Design review of the part built by this model. Coordinates are the model's own, in mm. A direction names the side the tool comes from. Coordinates: 2 decimals unless noted, no trailing zeros. Loops run counter-clockwise (first coordinate to the right, second up) from the corner with the lowest first, then second, coordinate; pieces in that order, holes last. Notation, with made-up numbers: (53, 54.5) - (105, 54.5) arc R22 cw to (105, 81.5) - close; hole circle Ø6 at (-34.5, 65.25). An arc over 180 degrees is marked (long way). One line per question, with ' | ' between items.
from build123d import *

# Parameters (mm, degrees)
SKETCH1_R           = 40
BOSS_EXTRUDE1_DEPTH = 4
SKETCH8_R           = 5
BOSS_EXTRUDE3_DEPTH = 5


with BuildPart() as part:
    # Sketch1 → Boss-Extrude1 (new body, symmetric)
    with BuildSketch(Plane(origin=(0, 0, 0), x_dir=(1, 0, 0), z_dir=(0, 1, 0))):
        Circle(SKETCH1_R)
    extrude(amount=BOSS_EXTRUDE1_DEPTH, both=True)

    # Sketch8 → Boss-Extrude3 (add)
    with BuildSketch(Plane(origin=(0, 0, 0), x_dir=(0, 0, -1), z_dir=(1, 0, 0))):
        with BuildLine():
            Line((0, 4), (-30, 4))
            Line((-30, 4), (37.824592442, 80.62784488))
            ThreePointArc((37.824592442, 80.62784488), (50.453649811, 82.577329326), (54.687857205, 70.520585679))
            Line((54.687857205, 70.520585679), (30, 4))
            Line((30, 4), (0, 4))
        make_face()
        with Locations((45.312694487, 74)):
            Circle(SKETCH8_R, mode=Mode.SUBTRACT)
    extrude(amount=BOSS_EXTRUDE3_DEPTH)


solid = part.part
Q1. Take a section at C-C (x = 3). Give the boundary of the cut face in (y, z).
Returned:
outline: (-4, -39.89) - (4, -39.89) - (4, -30) - (70.52, -54.69) arc R10 ccw to (80.63, -37.82) - (4, 30) - (4, 39.89) - (-4, 39.89) - close; hole circle Ø10 at (74, -45.31)
Q2. Take a section at B-B (y = 74). Give the boundary of the cut face in (x, z), plus the area to 3 significant figures.
Returned:
outline: (0, -55.31) - (5, -55.31) - (5, -50.31) - (0, -50.31) - close; (0, -40.31) - (5, -40.31) - (5, -31.96) - (0, -31.96) - close | area: 66.8 mm²
Q3. Take a section at A-A (z = -34.5). Give the boundary of the cut face in (x, y), plus the area to 3 significant figures.
Returned:
outline: (-20.24, -4) - (20.24, -4) - (20.24, 4) - (-20.24, 4) - close; (0, 16.13) - (5, 16.13) - (5, 76.87) - (0, 76.87) - close | area: 628 mm²
Q4. For pin 1 (10 mm diameter, centred on y = 15, z = -3, fed in from -X); pin 2 (8 mm diameter, centred on x = 5.5, y = 6.5, fed in from +Z); pin 3 (5 mm diameter, centred on x = 0.5, y = 7, fed in from +Z), all flat-tipped, find the tip position at first contact; note any pin that passes through.
Returned:
pin 1: stops at x = 0 | pin 2: stops at z = 39.93 | pin 3: stops at z = 29.56
Q5. To check wall thickness, follow line 1 along Y through (x, z) = (-8, -37); line 2 along X through (y, z) = (25.5, -15.5); line 3 along X through (y, z) = (2, -5). State the ranges of each line that lie inside material, in increasing order.
Returned:
line 1: y = -4 to 4 | line 2: x = 0 to 5 | line 3: x = -39.69 to 39.69
Q6. Tool access review of faces 4 (the flat face through (5, 36, -23)), 5 (the flat face through (0, 36, -23)), 6 (the flat face through (2.46, 37.73, -42.52)): name each direction out of +Z, -Z, +X, -X, +Y, -Y from which nothing blocks a thin tool from reaching the whole face with its end or side.
Returned:
face 4: +Z, -Z, +X, +Y | face 5: +Z, -Z, -X, +Y | face 6: -Z, +X, -X
Q7. Draft analysis for pull direction Z (two halves, no side actions). For faces 1 (the cylindrical face through (2.46, 69.12, -44.23)), 2 (the cylindrical face through (2.465, 82.675, -50.286)), 3 (the flat face through (-1, -4, -1)), state which applies: +Z half, -Z half, draft (parallel to the pull), parting line (faces both ways), or undercut.
Returned:
face 1: undercut | face 2: parting line | face 3: draft
Q8. Take a section at D-D (z = -2). Give the boundary of the cut face in (x, y).
Returned:
outline: (-39.95, -4) - (39.95, -4) - (39.95, 4) - (5, 4) - (5, 40.15) - (0, 40.15) - (0, 4) - (-39.95, 4) - close
